Build history of the part. All positions in model axes, mm. Face numbers are marked on the shaded views. A direction names the side the tool comes from. Give positions to 0.01 mm unless a question says otherwise; leave off trailing zeros. Order: outer loops, then holes, each group sorted by start corner. A loop starts at its lowest first (then second) coordinate and runs counter-clockwise, first axis right, second up. Notation, with made-up numbers: M 7.25,45 L 48.25,45 A8 ccw 48.25,51 Z; hole C 89,84.25 d11. An arc over 180 degrees is marked long. One line per item, written item: value. Start each with the question number.
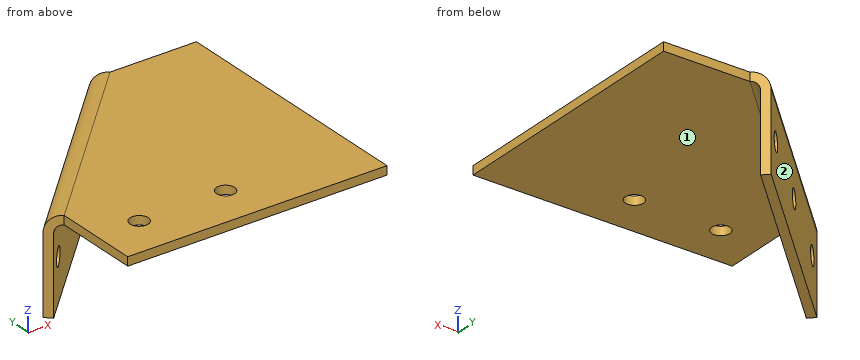
Autodesk Inventor part; units mm, degrees
ref_plane "YZ Plane" through (0, 0, 0) normal (1, 0, 0) x (0, 1, 0)
ref_plane "XZ Plane" through (0, 0, 0) normal (0, 1, 0) x (-1, 0, 0)
ref_plane "XY Plane" through (0, 0, 0) normal (0, 0, 1) x (1, 0, 0)
sketch "スケッチ1" plane through (0, 0, 0) normal (0, 0, 1) x (1, 0, 0)
  line L0 (0, 0) -> (80, 80)
  line L1 (80, 80) -> (80, 0)
  line L2 (80, 0) -> (0, 0)
  dimension "d0" = 45
  dimension "d1" = 80
extrude "プレート1" add sketch "スケッチ1" along normal blind 2
sketch "スケッチ2" plane through (0, 0, 2) normal (0, 0, 1) x (1, 0, 0)
  line L0 (0, 0) -> (80, 80)
  line L1 (0, 0) -> (20, 0)
  line L2 (20, 0) -> (20, 20)
  line L3 (20, 20) -> (0, 20)
  line L4 (0, 20) -> (0, 0)
  line L5 (80, 80) -> (60, 80)
  line L6 (60, 80) -> (60, 60)
  line L7 (60, 60) -> (80, 60)
  line L8 (80, 60) -> (80, 80)
  line L9 (0, 0) -> (80, 80)
  dimension "d3" = 20
  dimension "d6" = 20
extrude "押し出し1" cut sketch "スケッチ2" against normal blind 10 contours L0 L2 L1 | L6 L5 L0 | L0 L8 L7
sketch "スケッチ3" plane through (0, 0, 2) normal (0, 0, 1) x (1, 0, 0)
  line L0 (20, 20) -> (20, 0)
  line L1 (80, 0) -> (20, 0)
  line L2 (80, 60) -> (80, 0)
  line L3 (80, 60) -> (60, 60)
  line L4 (20, 20) -> (60, 60)
  line L5 (20, 20) -> (60, 60)
  line L6 (20, 20) -> (18.5858, 21.4142)
  line L7 (18.5858, 21.4142) -> (58.5858, 61.4142)
  line L8 (58.5858, 61.4142) -> (60, 60)
  point P0 (0, 0)
  dimension "d7" = 2
extrude "押し出し2" add sketch "スケッチ3" against normal up to surface (2 mm away) contours L6 L7 L8 L4
sketch "スケッチ4" plane through (58.5858, 61.4142, 0) normal (-0.7071068, 0.7071068, 0) x (-0.7071068, -0.7071068, 0)
  line L0 (56.5685, 0) -> (0, 0)
  line L1 (0, 0) -> (0, -20)
  line L2 (0, -20) -> (56.5685, -20)
  line L3 (56.5685, -20) -> (56.5685, 0)
edge flange "フランジ1" height 22 angle 90 thickness 2 bend radius 2 thickness toward (-0.7071068, 0.7071068, 0) relief tear relief width 2 relief depth 1 edges at (38.5858, 41.4142, 0) wall of the first edge with corners at (18.5858, 21.4142, 0) (58.5858, 61.4142, 0) (58.5858, 61.4142, -20) (18.5858, 21.4142, -20)
bend "曲げ1"
corner "コーナー1"
sketch "スケッチ5" plane through (18.5858, 21.4142, -2) normal (0.7071068, -0.7071068, 0) x (-0.7071068, -0.7071068, 0)
  line L0 (-56.5685, 0) -> (0, 0)
  line L1 (0, 0) -> (0, 18)
  line L2 (0, 18) -> (-56.5685, 18)
  line L3 (-56.5685, 0) -> (-56.5685, 18)
  line L4 (-56.5685, 0) -> (0, 0)
  point P0 (28.2843, -2)
  point P1 (-50.7843, 8)
  point P2 (-5.7843, 8)
  point P3 (-28.2843, 8)
  point P4 (-28.2843, 0)
  point P5 (-28.2843, 0)
  dimension "d20" = 10
  dimension "d23" = 45
  dimension "d24" = 22.5
hole "穴1" at (54.4957, 57.3241, -10) at (22.6759, 25.5043, -10) at (38.5858, 41.4142, -10) direction (-0.7071068, 0.7071068, 0) diameter 4.2 depth 2
sketch "スケッチ6" plane through (0, 0, 2) normal (0, 0, 1) x (1, 0, 0)
  line L0 (80, 0) -> (20, 0)
  line L1 (20, 20) -> (20, 0)
  line L2 (80, 60) -> (80, 0)
  point P0 (0, 0)
  point P1 (30, 10)
  point P2 (70, 10)
  point P3 (50, 10)
  dimension "d32" = 10
  dimension "d33" = 10
  dimension "d34" = 10
  dimension "d35" = 20
hole "穴2" at (30, 10, 2) at (50, 10, 2) direction (0, 0, -1) diameter 4.2 depth 2
equation "\"d30\" = Thickness"
equation "\"d41\" = Thickness"
equation "\"d2\" = Thickness"
equation "\"d10\" = BendReliefWidth"
equation "\"d11\" = BendReliefDepth"
equation "\"d12\" = MinimumRemnant"
equation "\"d13\" = TransitionRadius"
equation "\"d16\" = BendRadius"
equation "\"d17\" = CornerReliefSize"
equation "\"d18\" = GapSize"
equation "\"d19\" = JacobiRadiusSize"
equation "\"BendRadius\" = Thickness"
equation "\"BendReliefWidth\" = Thickness"
equation "\"BendReliefDepth\" = 0.5 * Thickness"
equation "\"CornerReliefSize\" = 4 * Thickness"
equation "\"MinimumRemnant\" = 2 * Thickness"
equation "\"TransitionRadius\" = BendRadius"
equation "\"JacobiRadiusSize\" = BendRadius"
equation "\"GapSize\" = Thickness"
properties part number "CoreXY_Angle"
1) Drill centre lines: line 1 (X direction, y = 10, z = 0.5); line 2 (Y direction, x = 50, z = 1); line 3 (Z direction, x = 61, y = 18). Where is each one in solid material? Low to high.
2) Slice it at B-B (z = -18.5). List the corners of the cut face in (x, y), plus the area to 3 significant figures.
3) Slice it at A-A (y = 10). List the corners of the cut face in (x, z), plus the area to 3 significant figures.
4) Tool access for the marked faces 1 and 2: list every direction of +Z, -Z, +X, -X, +Y, -Y with a clear straight run to the whole face (end or side of a thin tool).
5) Drop flat-ended pins along their axis: P1, Ø1, axis at y = 8.5, z = 0.5, coming from the -X side; P2, Ø6, axis at x = 36, z = -16.5, coming from the -Y side; P3, Ø2, axis at x = 45.5, z = -8.5, coming from the -Y side. Give the stop position or say it passes through.
Results list:
1. line 1: x = 20 to 27.9, 32.1 to 47.9, 52.1 to 80
1. line 2: y = 0 to 7.9, 12.1 to 53.74
1. line 3: z = 0 to 2
2. outline: M 17.17,22.83 L 18.59,21.41 L 58.59,61.41 L 57.17,62.83 Z
2. area: 113 mm²
3. outline: M 20,0 L 27.9,0 L 27.9,2 L 20,2 Z; M 32.1,0 L 47.9,0 L 47.9,2 L 32.1,2 Z; M 52.1,0 L 80,0 L 80,2 L 52.1,2 Z
3. area: 103 mm²
4. face 1: -Z, +X, -Y
4. face 2: +Z, -Z, -X, +Y
5. P1: stops at x = 20
5. P2: stops at y = 35.83
5. P3: stops at y = 47.33
